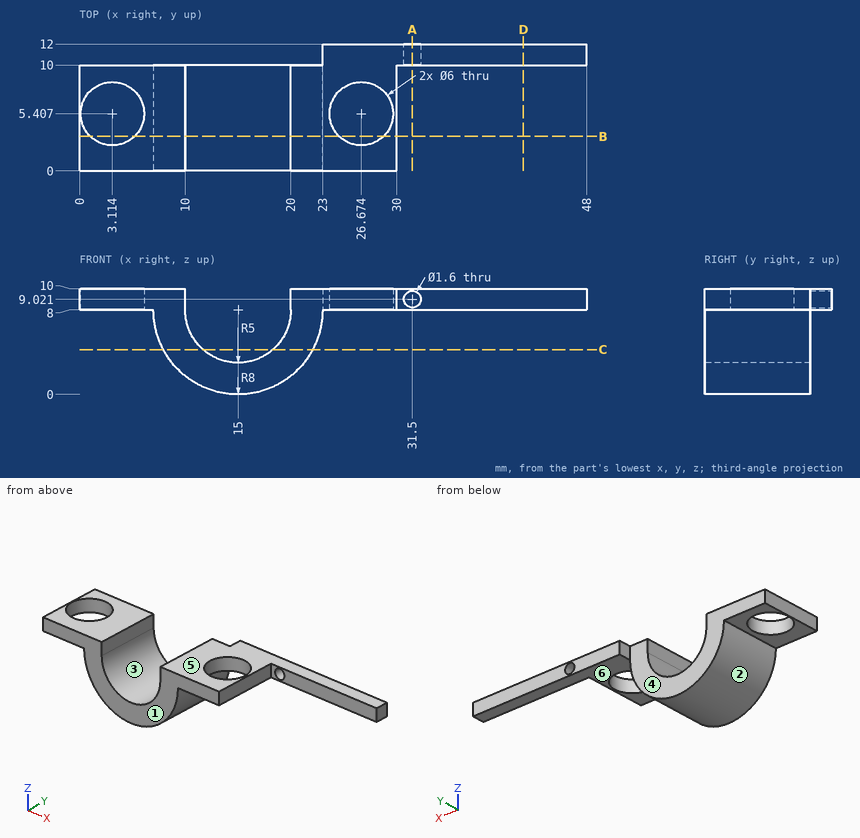
Part print with two shaded views. Sizes in mm from the minimum x, y, z corner. A direction names the side the tool comes from. Coordinates: 2 decimals unless noted, no trailing zeros. Order: outer loops, then holes, each group sorted by start corner. A loop starts at its lowest first (then second) coordinate and runs counter-clockwise, first axis right, second up.
(1) Drill centre lines: L1, parallel to Z at x = 31.5, y = 11.3; L2, parallel to X at y = 3.5, z = 8.5; L3, parallel to Y at x = 11, z = 1.25. Where is each one in solid material? Low to high.
Solution:
L1: z = 8 to 8.22, 9.82 to 10
L2: x = 0 to 0.8, 5.43 to 10, 20 to 24.36, 28.99 to 30
L3: y = 0 to 10
(2) Saw through at C-C, the plane z = 4.25. Write the cut outline in (x, y).
Solution:
outline: (7.93, 0) - (11.69, 0) - (11.69, 10) - (7.93, 10) - close; (18.31, 0) - (22.07, 0) - (22.07, 10) - (18.31, 10) - close
(3) Saw through at D-D, the plane x = 42. Write the cut outline in (y, z), and give its area (3 significant figures).
Solution:
outline: (10, 8) - (12, 8) - (12, 10) - (10, 10) - close
area: 4.00 mm2
(4) Which spindle directions (+Z, -Z, +X, -X, +Y, -Y) get a long thin tool onto all of the face, cutting with end or side? Do the marked faces 4, 5 and 6. Say none if no direction does.
Solution:
face 4: +Z, -Z, -X, +Y
face 5: +Z, +X, -X, +Y, -Y
face 6: -Z, +X, +Y, -Y
(5) Saw through at B-B, the plane y = 3.25. Write the cut outline in (x, z).
Solution:
outline: (0, 8) - (1.03, 8) - (1.03, 10) - (0, 10) - close; (5.2, 8) - (7, 8) arc R8 ccw to (23, 8) - (24.59, 8) - (24.59, 10) - (20, 10) - (20, 8) arc R5 cw to (10, 8) - (10, 10) - (5.2, 10) - close; (28.76, 8) - (30, 8) - (30, 10) - (28.76, 10) - close
(6) Saw through at A-A, the plane x = 31.5. Write the cut outline in (y, z).
Solution:
outline: (10, 8) - (12, 8) - (12, 8.22) - (10, 8.22) - close; (10, 9.82) - (12, 9.82) - (12, 10) - (10, 10) - close
(7) Pin check, flat tips, straight feed: pin 1 Ø2 at (x, z) = (31.5, 9.02) entering from -Y; pin 2 Ø3 at (y, z) = (5, 4.5) entering from -X; pin 3 Ø2 at (y, z) = (4, 9.5) entering from +X. Stop position of each tip, or through.
Solution:
pin 1: stops at y = 10
pin 2: stops at x = 7.25
pin 3: stops at x = 30
(8) Mould opens along X. For the marked faces 1, 2 and 3 say: released by +X, released by -X, zero draft, split by the parting line, or undercut.
Solution:
face 1: zero draft
face 2: split by the parting line
face 3: undercut
